Here's how the part is built. I have some questions about the finished solid (model axes, mm). A direction names the side the tool comes from. Give positions to 0.01 mm unless a question says otherwise; leave off trailing zeros. Order: outer loops, then holes, each group sorted by start corner. A loop starts at its lowest first (then second) coordinate and runs counter-clockwise, first axis right, second up. Notation, with made-up numbers: M 5.5,-2.5 L 26.5,-2.5 A23 ccw 26.5,8.5 Z; hole C 9.5,88 d3. An arc over 180 degrees is marked long. One line per item, written item: value. Start each with the question number.
from build123d import *

# Parameters (mm, degrees)
F1_DEPTH = 300
F3_DEPTH = 60.001
F5_DEPTH = 60.001


with BuildPart() as f1:
    # F0 (on Front) → F1 (new body)
    with BuildSketch(Plane.XZ):
        Polygon((60, 0), (0, 0), (0, -60), (2.5, -60), (2.5, -2.5), (60, -2.5), align=None)
    extrude(amount=F1_DEPTH)

    # F2 (on face) → F3 (cut, through all)
    with BuildSketch(Plane(origin=(0, 0, 0), x_dir=(0, -1, 0), z_dir=(-1, 0, 0))):
        Polygon((0, 0), (0, -60), (60, -60), align=None)
    extrude(amount=-F3_DEPTH, mode=Mode.SUBTRACT)

    # F4 (on face) → F5 (cut, through all)
    with BuildSketch(Plane(origin=(0, 0, 0), x_dir=(0, -1, 0), z_dir=(-1, 0, 0))):
        Polygon((240, 0), (300, -60), (300, 0), align=None)
    extrude(amount=-F5_DEPTH, mode=Mode.SUBTRACT)


solid = f1.part
Item 1: I want a section at B-B on x = 53. Write out the boundary of the cut face in (y, z).
Item 2: I want a section at A-A on y = -139.5. Write out the boundary of the cut face in (x, z), plus the area to 3 significant figures.
Item 3: Will these pins go through, and if not, where does the flat tip stop? P1, Ø12, axis at x = 18.5, y = -155.5, coming from the -Z side; P2, Ø1.5, axis at y = -64.5, z = -8.5, coming from the +X side.
Item 4: I want a section at D-D on y = -42.5. Write out the boundary of the cut face in (x, z), plus the area to 3 significant figures.
Item 5: For faces 1 (the face through (31, -121, -2.5)), 2 (the face through (1, -17, -17)), which set-ups out of +Z, -Z, +X, -X, +Y, -Y let a thin tool reach every point of the face, with its end or its side?
Item 6: I want a section at C-C on z = -25. Write out the boundary of the cut face in (x, y), plus the area to 3 significant figures.
Item 7: Please list where these lines run through material, in increasing order: probe 1 along X at (y, z) = (-59.5, -45.5); probe 2 along Z at (x, y) = (24, -169.5); probe 3 along Z at (x, y) = (28.5, -241). Write a range as [from, to].
Answer below:
1. outline: M -242.5,-2.5 L -2.5,-2.5 L 0,0 L -240,0 Z
2. outline: M 0,-60 L 2.5,-60 L 2.5,-2.5 L 60,-2.5 L 60,0 L 0,0 Z
2. area: 294 mm²
3. P1: stops at z = -2.5
3. P2: stops at x = 2.5
4. outline: M 0,-42.5 L 2.5,-42.5 L 2.5,-2.5 L 60,-2.5 L 60,0 L 0,0 Z
4. area: 250 mm²
5. face 1: -Z, +X, +Y, -Y
5. face 2: -Z, +X, -X, +Y
6. outline: M 0,-265 L 2.5,-265 L 2.5,-25 L 0,-25 Z
6. area: 600 mm²
7. probe 1: x = [0, 2.5]
7. probe 2: z = [-2.5, 0]
7. probe 3: z = [-2.5, -1]
